Read the model definition and answer for the solid it produces. Units are mm, in the model's axes. A direction names the side the tool comes from. Coordinates: 2 decimals unless noted, no trailing zeros. Loops run counter-clockwise (first coordinate to the right, second up) from the corner with the lowest first, then second, coordinate; pieces in that order, holes last. Notation, with made-up numbers: (-28, 36) - (17, 36) arc R15 ccw to (17, 50) - close; hole circle Ø3 at (84.25, 63). An arc over 180 degrees is marked (long way). Use CSV: the item, a comma, the result in double quotes.
```python
from build123d import *

# Parameters (mm, degrees)
SKETCH1_W           = 60
SKETCH1_H           = 30
SKETCH1_R           = 9
SKETCH1_R_2         = 5
BOSS_EXTRUDE1_DEPTH = 10
FILLET1_R           = 8
SKETCH1_3_R         = 9
SKETCH1_3_R_2       = 5
BOSS_EXTRUDE2_DEPTH = 25


with BuildPart() as part:
    # Sketch1 → Boss-Extrude1 (new body)
    # profile 1 of 2: a face of its own
    with BuildSketch(Plane(origin=(0, 0, 0), x_dir=(1, 0, 0), z_dir=(0, 1, 0))):
        with Locations((-21, 0)):
            Rectangle(SKETCH1_W, SKETCH1_H)
        Circle(SKETCH1_R, mode=Mode.SUBTRACT)
    # profile 2 of 2: a face of its own
    with BuildSketch(Plane(origin=(0, 0, 0), x_dir=(1, 0, 0), z_dir=(0, 1, 0))):
        Circle(SKETCH1_R)
        with Locations(Location((0, 0, 0), (0, 0, 270))):
            Circle(SKETCH1_R_2, mode=Mode.SUBTRACT)
    extrude(amount=BOSS_EXTRUDE1_DEPTH)

    # Fillet1
    fillet1_edges = [part.edges().sort_by_distance(p)[0] for p in [
        (9, 5, 15),
        (-51, 5, 15),
        (-51, 5, -15),
        (9, 5, -15),
    ]]
    fillet(fillet1_edges, radius=FILLET1_R)

    # Sketch1_3 → Boss-Extrude2 (add)
    with BuildSketch(Plane(origin=(0, 0, 0), x_dir=(1, 0, 0), z_dir=(0, 1, 0))):
        Circle(SKETCH1_3_R)
        with Locations(Location((0, 0, 0), (0, 0, 270))):
            Circle(SKETCH1_3_R_2, mode=Mode.SUBTRACT)
    extrude(amount=BOSS_EXTRUDE2_DEPTH)


solid = part.part
```
Q1. The part is cut by section D-D on z = 11.5. Determine the outline of the cut face in (x, y).
Reported:
outline,"(-49.61, 0) - (7.61, 0) - (7.61, 10) - (-49.61, 10) - close"
Q2. The part is cut by section A-A on x = 0. Determine the outline of the cut face in (y, z).
Reported:
outline,"(0, -15) - (10, -15) - (10, -9) - (25, -9) - (25, -5) - (0, -5) - close; (0, 5) - (25, 5) - (25, 9) - (10, 9) - (10, 15) - (0, 15) - close"
Q3. Given P1, Ø4, axis at y = 16.5, z = 10, coming from the +X side; P2, Ø10, axis at y = 21, z = 3.5, coming from the -X side; P3, Ø6, axis at x = -20, y = 15.5, coming from the -Z side; P4, Ø5, axis at y = 21.5, z = -7.5, coming from the +X side, each flat-ended and moving along its own axis, determine where each tip first touches the part or whether it passes through.
Reported:
P1,"stops at x = 4.12"
P2,"stops at x = -9"
P3,"passes through"
P4,"stops at x = 7.48"
Q4. The part is cut by section C-C on x = -21.5. Determine the outline of the cut face in (y, z).
Reported:
outline,"(0, -15) - (10, -15) - (10, 15) - (0, 15) - close"
Q5. The part is cut by section B-B on y = 7.25. Determine the outline of the cut face in (x, z), and give its area (3 significant figures).
Reported:
outline,"(-51, -7) arc R8 ccw to (-43, -15) - (1, -15) arc R8 ccw to (9, -7) - (9, 7) arc R8 ccw to (1, 15) - (-43, 15) arc R8 ccw to (-51, 7) - close; hole circle Ø10 at (0, 0)"
area,"1,670 mm²"
Q6. A tool of negligible diameter and unlimited length cuts with its end or side. For faces 4 (the face through (-1.172, 17.395, -8.923)), 5 (the face through (4, 25, 4)), from which of +Z, -Z, +X, -X, +Y, -Y can it reach the whole face along a straight path? Write none if from no direction.
Reported:
face 4,"+Y"
face 5,"+Z, -Z, +X, -X, +Y"
Q7. Find the intervals of material crossed by probe 1 along X at (y, z) = (16, 0); probe 2 along Y at (x, z) = (-10, 7); probe 3 along X at (y, z) = (23.5, 1.5), in increasing order. Write a range as [from, to].
Reported:
probe 1,"x = [-9, -5], [5, 9]"
probe 2,"y = [0, 10]"
probe 3,"x = [-8.87, -4.77], [4.77, 8.87]"
Q8. For a pull along X with two mould halves and no side action, classify faces 1 (the face through (-48.594, 5.07, -12.719)), 2 (the face through (-4.88, 12.32, -1.08)), 3 (the face through (-21, 5, 15)) as +X half, -X half, draft (parallel to the pull), parting line (faces both ways), or undercut.
Reported:
face 1,"-X half"
face 2,"undercut"
face 3,"draft"
